Design review of the part built by this model. Coordinates are the model's own, in mm. A direction names the side the tool comes from. Round coordinates to 2 decimals unless told otherwise and drop trailing zeros. Order: outer loops, then holes, each group sorted by start corner. A loop starts at its lowest first (then second) coordinate and runs counter-clockwise, first axis right, second up. Notation, with made-up numbers: M 87,30.5 L 143,30.5 A10 ccw 143,43.5 Z; hole C 18,-4.5 d11. An arc over 180 degrees is marked long. Write item = value, one per line. Start each with the question number.
Autodesk Inventor part; units mm, degrees
ref_plane "YZ Plane" through (0, 0, 0) normal (1, 0, 0) x (0, 1, 0)
ref_plane "XZ Plane" through (0, 0, 0) normal (0, 1, 0) x (-1, 0, 0)
ref_plane "XY Plane" through (0, 0, 0) normal (0, 0, 1) x (1, 0, 0)
sketch "Sketch1" plane through (0, 0, 0) normal (0, 1, 0) x (-1, 0, 0)
  line L0 (0, 0) -> (100, 0)
  line L1 (100, 0) -> (100, -100)
  line L2 (100, -100) -> (0, -100)
  line L3 (0, -100) -> (0, 0)
  dimension "d0" = 100
  dimension "d1" = 100
extrude "Extrusion1" add sketch "Sketch1" along normal blind 5
sketch "Sketch2" plane through (0, 5, 0) normal (0, 1, 0) x (1, 0, 0)
  line L0 (0, 100) -> (-100, 100)
  line L1 (-100, 100) -> (-100, 0)
  line L2 (-100, 0) -> (0, 0)
  line L3 (0, 0) -> (0, 100)
  line L4 (-58.25, 37.25) -> (-41.75, 37.25)
  line L5 (-41.75, 37.25) -> (-41.75, 62.75)
  line L6 (-41.75, 62.75) -> (-58.25, 62.75)
  line L7 (-58.25, 62.75) -> (-58.25, 37.25)
  line L8 (-66.25, 29.25) -> (-33.75, 29.25)
  line L9 (-33.75, 29.25) -> (-33.75, 70.75)
  line L10 (-33.75, 70.75) -> (-66.25, 70.75)
  line L11 (-66.25, 70.75) -> (-66.25, 29.25)
  line L12 (-100, 100) -> (-100, 0) construction
  line L13 (0, 100) -> (-100, 100) construction
  line L14 (-100, 0) -> (0, 100) construction
  line L15 (0, 100) -> (-100, 100) construction
  line L16 (-100, 100) -> (0, 0) construction
  line L17 (-66.25, 29.25) -> (-33.75, 70.75) construction
  line L18 (-66.25, 70.75) -> (-33.75, 29.25) construction
  point P0 (-50, 50)
  dimension "d7" = 16.5
  dimension "d8" = 25.5
  dimension "d10" = 8
extrude "Extrusion2" add sketch "Sketch2" along normal blind 15 contours L11 L10 L9 L8
sketch "Sketch3" plane through (0, 5, 0) normal (0, 1, 0) x (1, 0, 0)
  line L0 (-58.25, 37.25) -> (-41.75, 37.25)
  line L1 (-41.75, 37.25) -> (-41.75, 62.75)
  line L2 (-41.75, 62.75) -> (-58.25, 62.75)
  line L3 (-58.25, 62.75) -> (-58.25, 37.25)
  point P0 (0, 0)
extrude "Extrusion3" add sketch "Sketch3" along normal blind 5
sketch "Sketch4" plane through (0, 10, 0) normal (0, 1, 0) x (1, 0, 0)
  line L0 (-41.75, 62.75) -> (-41.75, 37.25)
  line L1 (-58.25, 62.75) -> (-41.75, 62.75)
  line L2 (-58.25, 37.25) -> (-58.25, 62.75)
  line L3 (-41.75, 37.25) -> (-58.25, 37.25)
  line L4 (-58.25, 37.25) -> (-41.75, 62.75) construction
  line L5 (-58.25, 62.75) -> (-41.75, 37.25) construction
  circle A0 centre (-50, 50) radius 2.75
  point P0 (0, 0)
  dimension "d15" = 5.5
extrude "Extrusion4" cut sketch "Sketch4" against normal through all contours A0
sketch "Sketch5" plane through (0, 0, 0) normal (0, -1, 0) x (1, 0, 0)
  circle A0 centre (-50, -50) radius 2.75
  line L0 (0, -100) -> (-100, -100)
  line L1 (0, 0) -> (0, -100)
  line L2 (-100, 0) -> (0, 0)
  line L3 (-100, -100) -> (-100, 0)
  circle A1 centre (-50, -50) radius 4.5
  dimension "d18" = 9
extrude "Extrusion5" cut sketch "Sketch5" against normal blind 5.5 contours A0 | A1
fillet "Fillet1" radius 5 4 edges at (-66.25, 5, -50) (-50, 5, -70.75) (-50, 5, -29.25) (-33.75, 5, -50)
fillet "Fillet2" radius 2 20 edges at (-33.75, 20, -50) (-50, 20, -70.75) (-66.25, 20, -50) (-50, 20, -29.25) (-67.7145, 6.4645, -27.7855) (-66.25, 15, -29.25) (-67.7145, 6.4645, -72.2145) (-66.25, 15, -70.75) (-32.2855, 6.4645, -27.7855) (-33.75, 15, -29.25) (-32.2855, 6.4645, -72.2145) (-33.75, 15, -70.75) (0, 5, -50) (-50, 5, 0) (0, 2.5, 0) (-50, 5, -100) (0, 2.5, -100) (-100, 2.5, -100) (-100, 5, -50) (-100, 2.5, 0)
chamfer "Chamfer1" distance 1 angle 45 4 edges at (-58.25, 20, -50) (-50, 20, -62.75) (-50, 20, -37.25) (-41.75, 20, -50)
properties part number "base_frame"
(1) For line 1 along Z through (x, y) = (-50, 1.65); line 2 along Z through (x, y) = (-40, 10.75); line 3 along X through (y, z) = (7.1, -50), list the stretches that pass through material, from the lowest coordinate up. Write a range as [from, to].
(2) Consider section B-B, the plane z = -50. Write out the cut boundary in (x, y).
(3) Consider section C-C, the plane y = 14.5. Write out the cut boundary in (x, z), then the cut area to 3 significant figures.
(4) Draft analysis for pull direction Z (two halves, no side actions). For faces 5 (the face through (-51, 1, -100)), 6 (the face through (-50, 14, -37.25)), 7 (the face through (-32.25, 6.43, -50.36)), state which applies: pulls with the +Z half, pulls with the -Z half, needs draft (parallel to the pull), parting line crosses it, or undercut.
(5) Consider section D-D, the plane z = -15.5. Write out the cut boundary in (x, y), then the cut area to 3 significant figures.
(6) For faces 1 (the face through (-50, 10, -53)), 2 (the face through (-50, 5.5, -53)), 3 (the face through (-50, 14, -70.75)), 4 (the face through (-66.25, 14, -50)), list the 3-axis set-ups (+Z, -Z, +X, -X, +Y, -Y) from which the entire face can be reached by the end or side of a thin tool; tool diameter is ignored.
(7) Insertion check: pin 1 (10 mm diameter, centred on x = -42, z = -38.5, fed in from +Y); pin 2 (2.5 mm diameter, centred on y = 14.5, z = -54, fed in from -X); pin 3 (9 mm diameter, centred on y = 16, z = -52.5, fed in from +X); pin 4 (5 mm diameter, centred on y = 7, z = -27, fed in from -X). Each pin has a flat end and moves straight along its axis. Give the tip position at first contact, or say it passes through.
(8) Consider section A-A, the plane x = -50. Write out the cut boundary in (y, z).
Completed:
q1.line_1 = [-100, -54.5], [-45.5, 0]
q1.line_2 = [-70.75, -29.25]
q1.line_3 = [-67.18, -52.75], [-47.25, -32.82]
q2.outline = M -100,0 L -54.5,0 L -54.5,5.5 L -52.75,5.5 L -52.75,10 L -58.25,10 L -58.25,19 L -59.25,20 L -64.25,20 A2 ccw -66.25,18 L -66.25,10 A5 cw -71.25,5 L -98,5 A2 ccw -100,3 Z; M -47.25,5.5 L -45.5,5.5 L -45.5,0 L 0,0 L 0,3 A2 ccw -2,5 L -28.75,5 A5 cw -33.75,10 L -33.75,18 A2 ccw -35.75,20 L -40.75,20 L -41.75,19 L -41.75,10 L -47.25,10 Z
q3.outline = M -66.25,-68.75 A2 ccw -64.25,-70.75 L -35.75,-70.75 A2 ccw -33.75,-68.75 L -33.75,-31.25 A2 ccw -35.75,-29.25 L -64.25,-29.25 A2 ccw -66.25,-31.25 Z; hole M -58.25,-62.75 L -41.75,-62.75 L -41.75,-37.25 L -58.25,-37.25 Z
q3.area = 925 mm2
q4.face_5 = pulls with the -Z half
q4.face_6 = undercut
q4.face_7 = needs draft
q5.outline = M -100,0 L 0,0 L 0,3 A2 ccw -2,5 L -98,5 A2 ccw -100,3 Z
q5.area = 498 mm2
q6.face_1 = +Y
q6.face_2 = -Y
q6.face_3 = -Z, +X, -X, +Y
q6.face_4 = +Z, -Z, -X, +Y
q7.pin_1 = 20
q7.pin_2 = -66.25
q7.pin_3 = -33.75
q7.pin_4 = -99.32
q8.outline = M 0,-100 L 3,-100 A2 ccw 5,-98 L 5,-75.75 A5 cw 10,-70.75 L 18,-70.75 A2 ccw 20,-68.75 L 20,-63.75 L 19,-62.75 L 10,-62.75 L 10,-52.75 L 5.5,-52.75 L 5.5,-54.5 L 0,-54.5 Z; M 0,-45.5 L 5.5,-45.5 L 5.5,-47.25 L 10,-47.25 L 10,-37.25 L 19,-37.25 L 20,-36.25 L 20,-31.25 A2 ccw 18,-29.25 L 10,-29.25 A5 cw 5,-24.25 L 5,-2 A2 ccw 3,0 L 0,0 Z
